Input: part model. Units: mm. Frame: model coordinates. Face numbers are marked on the shaded views. A direction names the side the tool comes from. Give positions to 0.01 mm unless a question says otherwise; leave off trailing zeros. Write each loop counter-clockwise with the first axis right and the second up, starting at its lowest first coordinate (ties: lowest second). Pieces come first, ordered by that corner, then holes. Notation, with made-up numbers: (-13, 50) - (-6, 50) arc R27 cw to (-6, 84) - close; hole circle Ø10 at (-24.75, 38). An arc over 180 degrees is marked (long way). Answer as a JSON object with one key per item and string values. Group by question number.
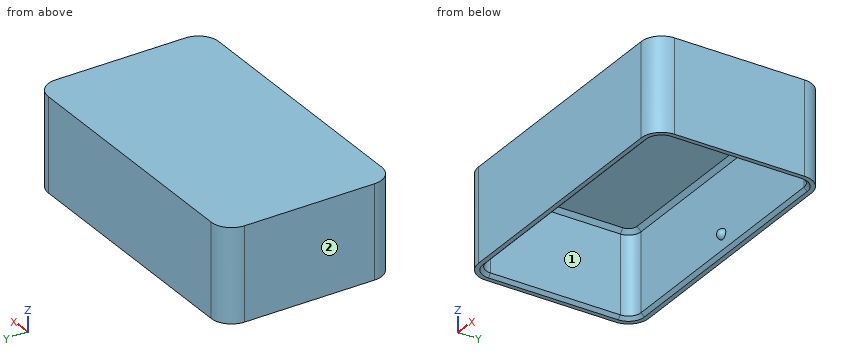
from build123d import *

# Parameters (mm, degrees)
F0_W     = 72
F0_H     = 42
F1_DEPTH = 23
F2_R     = 5
F3_T     = -1.9
F4_SIZE  = 0.8
F5_SIZE  = 1


with BuildPart() as f1:
    # F0 (on Top) → F1 (new body)
    with BuildSketch(Plane.XY):
        Rectangle(F0_W, F0_H)
    extrude(amount=F1_DEPTH)

    # F2
    f2_edges = [f1.edges().sort_by_distance(p)[0] for p in [
        (-36, -21, 11.5),
        (36, -21, 11.5),
        (36, 21, 11.5),
        (-36, 21, 11.5),
    ]]
    fillet(f2_edges, radius=F2_R)

    # F3
    f3_openings = [f1.faces().sort_by_distance(p)[0] for p in [
        (0, 0, 0),
    ]]
    offset(amount=F3_T, openings=f3_openings)

    # F4
    f4_edges = [f1.edges().sort_by_distance(p)[0] for p in [
        (34.1, 0, 0),
        (33.192031, -18.192031, 0),
        (0, -19.1, 0),
        (-33.192031, -18.192031, 0),
        (-34.1, 0, 0),
        (-33.192031, 18.192031, 0),
        (0, 19.1, 0),
        (33.192031, 18.192031, 0),
    ]]
    chamfer(f4_edges, length=F4_SIZE)

    # F5
    f5_edges = [f1.edges().sort_by_distance(p)[0] for p in [
        (34.1, 0, 21.1),
        (33.192031, 18.192031, 21.1),
        (0, 19.1, 21.1),
        (-33.192031, 18.192031, 21.1),
        (-34.1, 0, 21.1),
        (-33.192031, -18.192031, 21.1),
        (0, -19.1, 21.1),
        (33.192031, -18.192031, 21.1),
    ]]
    chamfer(f5_edges, length=F5_SIZE)

    # F7 (on offset) → F8 (revolve)
    with BuildSketch(Plane(origin=(0, 0, 4.5), x_dir=(1, 0, 0), z_dir=(0, 0, -1))):
        with BuildLine():
            Line((0, -19.1), (1.25, -19.1))
            ThreePointArc((1.25, -19.1), (0.8838834765, -18.2161165235), (0, -17.85))
            Line((0, -17.85), (0, -19.1))
        make_face()
        with BuildLine():
            Line((0, 19.1), (-1.25, 19.1))
            ThreePointArc((-1.25, 19.1), (-0.8838834765, 18.2161165235), (0, 17.85))
            Line((0, 17.85), (0, 19.1))
        make_face()
    revolve(axis=Axis((0, 18.475, 4.5), (0, 1, 0)))


solid = f1.part
1) Reachability of the marked faces 1 and 2 from +Z, -Z, +X, -X, +Y, -Y: full face, straight path, thin tool, end or side. Return the list, or none.
2) Line query: line 1 along Y through (x, z) = (-0.5, 7); line 2 along X through (y, z) = (0.5, 11.5); line 3 along Z through (x, y) = (-15, -8.5). Output: solid intervals per line, ascending. Write a range as from..to.
3) Cut plane C-C on y = 14. Return the cut outline in (x, z), and give its area (3 significant figures).
4) Cut plane A-A on z = 6.5. Return the cut outline in (x, y), and give its area (3 significant figures).
5) Cut plane B-B on x = -14. Return the cut outline in (y, z), and give its area (3 significant figures).
6) Pin query (flat end, axial travel): P1, Ø18, axis at x = -12.5, y = -5, coming from the -Z side. Return the tip coordinate at first contact, or that it passes through.
Filled in:
{
 "1": {"face 1": "-Z", "face 2": "+Z, -Z, -X, +Y, -Y"},
 "2": {"line 1": "y = -21..-19.1, 19.1..21", "line 2": "x = -36..-34.1, 34.1..36", "line 3": "z = 21.1..23"},
 "3": {"outline": "(-36, 0) - (-34.9, 0) - (-34.1, 0.8) - (-34.1, 20.1) - (-33.1, 21.1) - (33.1, 21.1) - (34.1, 20.1) - (34.1, 0.8) - (34.9, 0) - (36, 0) - (36, 23) - (-36, 23) - close", "area": "217 mm²"},
 "4": {"outline": "(-36, -16) arc R5 ccw to (-31, -21) - (31, -21) arc R5 ccw to (36, -16) - (36, 16) arc R5 ccw to (31, 21) - (-31, 21) arc R5 ccw to (-36, 16) - close; hole (-34.1, -16) arc R3.1 ccw to (-31, -19.1) - (31, -19.1) arc R3.1 ccw to (34.1, -16) - (34.1, 16) arc R3.1 ccw to (31, 19.1) - (-31, 19.1) arc R3.1 ccw to (-34.1, 16) - close", "area": "406 mm²"},
 "5": {"outline": "(-21, 0) - (-19.9, 0) - (-19.1, 0.8) - (-19.1, 20.1) - (-18.1, 21.1) - (18.1, 21.1) - (19.1, 20.1) - (19.1, 0.8) - (19.9, 0) - (21, 0) - (21, 23) - (-21, 23) - close", "area": "160 mm²"},
 "6": {"P1": "stops at z = 21.1"}
}
